CAD build for the part. Positions are in the model's coordinates, mm. Face numbers are marked on the shaded views. Give positions to 0.01 mm unless a question says otherwise; leave off trailing zeros. Loops run counter-clockwise (first coordinate to the right, second up) from the corner with the lowest first, then second, coordinate; pieces in that order, holes last. Notation, with made-up numbers: (48, 7.25) -> (98, 7.25) arc R10 ccw to (98, 15.25) -> close; hole circle Ø10 at (50, 58.25). An arc over 180 degrees is marked (long way). Use one line per item in the form item = value.
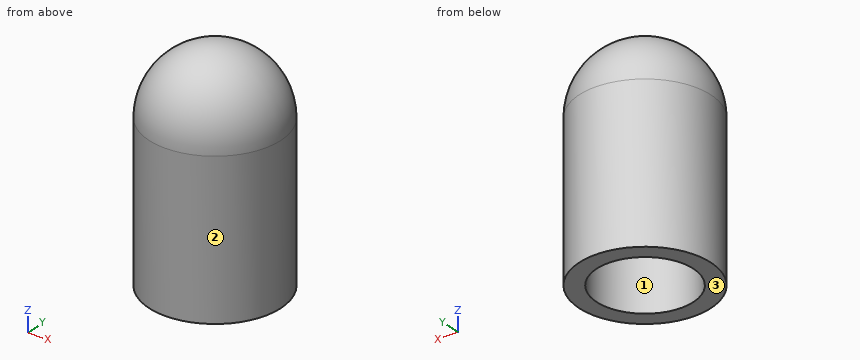
```python
from build123d import *

# Parameters (mm, degrees)
F0_R     = 7.5
F1_DEPTH = 25
F3_D     = 5
F3_DEPTH = 20
F3_TIP   = 1.5021515476
F5_D     = 11
F5_DEPTH = 11
F5_TIP   = 3.3047334047
F6_R     = 7.5


with BuildPart() as f1:
    # F0 (on Top) → F1 (new body)
    with BuildSketch(Plane.XY):
        Circle(F0_R)
    extrude(amount=F1_DEPTH)

    # F3
    with Locations(Plane(origin=(0, 0, 0), x_dir=(1, 0, 0), z_dir=(0, 0, -1))):
        with Locations((0, 0)):
            Hole(F3_D / 2, depth=F3_DEPTH)
            with Locations((0, 0, -(F3_DEPTH + F3_TIP / 2))):  # 118° drill point
                Cone(0, F3_D / 2, F3_TIP, mode=Mode.SUBTRACT)

    # F5
    with Locations(Plane(origin=(0, 0, 0), x_dir=(1, 0, 0), z_dir=(0, 0, -1))):
        with Locations((0, 0)):
            Hole(F5_D / 2, depth=F5_DEPTH)
            with Locations((0, 0, -(F5_DEPTH + F5_TIP / 2))):  # 118° drill point
                Cone(0, F5_D / 2, F5_TIP, mode=Mode.SUBTRACT)

    # F6
    f6_edges = [f1.edges().sort_by_distance(p)[0] for p in [
        (-7.5, 0, 25),
    ]]
    fillet(f6_edges, radius=F6_R)


solid = f1.part
```
1. Drop flat-ended pins along their axis: P1, Ø3, axis at x = 0, y = 0, coming from the -Z side; P2, Ø3, axis at x = -1.5, y = -3, coming from the -Z side; P3, Ø5, axis at x = 5.5, z = 13, coming from the +Y side; P4, Ø8, axis at x = 3.5, z = 10, coming from the -Y side. Give the stop position or say it passes through.
Result sheet:
P1 = 20.6
P2 = 11.39
P3 = 6.87
P4 = -7.5
2. Cut at B-B, the plane z = 3.25. Write the cut outline in (x, y), then the cut area to 3 significant figures.
Result sheet:
outline = circle Ø15 at (0, 0); hole circle Ø11 at (0, 0)
area = 81.7 mm^2
3. Cut at A-A, the plane z = 17. Write the cut outline in (x, y).
Result sheet:
outline = circle Ø15 at (0, 0); hole circle Ø5 at (0, 0)
4. Drill centre lines: line 1 (Y direction, x = 0, z = 7.75); line 2 (X direction, y = -0.75, z = 16.25); line 3 (X direction, y = 1.75, z = 12.5). Where is each one in solid material? Low to high.
Result sheet:
line_1 = -7.5 to -5.5, 5.5 to 7.5
line_2 = -7.46 to -2.38, 2.38 to 7.46
line_3 = -7.29 to -2.44, 2.44 to 7.29
5. Mould opens along X. For the marked faces 1, 2 and 3 say: pulls with the +X half, pulls with the -X half, needs draft (parallel to the pull), parting line crosses it, or undercut.
Result sheet:
face_1 = undercut
face_2 = parting line crosses it
face_3 = needs draft
